```python
from build123d import *

# Parameters (mm, degrees)
BOSS_EXTRUDE1_DEPTH = 50
SKETCH2_W           = 100
SKETCH2_H           = 5
BOSS_EXTRUDE2_DEPTH = 80


with BuildPart() as part:
    # Sketch1 → Boss-Extrude1 (new body)
    with BuildSketch(Plane(origin=(0, 0, 0), x_dir=(1, 0, 0), z_dir=(0, 1, 0))):
        Polygon((0, 0), (490, 0), (490, 20), (420, 20), (420, 170), (400, 170), (400, 20), (310, 20), (310, 170), (290, 170), (290, 20), (200, 20), (200, 170), (180, 170), (180, 20), (90, 20), (90, 170), (70, 170), (70, 20), (0, 20), align=None)
    extrude(amount=BOSS_EXTRUDE1_DEPTH)

    # Sketch2 → Boss-Extrude2 (add)
    with BuildSketch(Plane.XY):
        with Locations((50, 2.5)):
            Rectangle(SKETCH2_W, SKETCH2_H)
    extrude(amount=BOSS_EXTRUDE2_DEPTH)


solid = part.part
```
Read the model definition and answer for the solid it produces. Units are mm, in the model's axes. A direction names the side the tool comes from. Give positions to 0.01 mm unless a question says otherwise; leave off trailing zeros. Write each loop counter-clockwise with the first axis right and the second up, starting at its lowest first coordinate (ties: lowest second). Pieces come first, ordered by that corner, then holes. Notation, with made-up numbers: M -20.5,14.5 L -1.5,14.5 A16 ccw -1.5,39.5 Z; hole C -31,68.25 d9. An arc over 180 degrees is marked long. Put each result on its own line as item: value. Start each with the question number.
1. Consider line 1 along X through (y, z) = (27, -58.5); line 2 along Z through (x, y) = (94, 24.5); line 3 along Z through (x, y) = (24, 4). Determine where each line is inside the solid, lowest interval first.
2. The part is cut by section D-D, the plane z = 56.5. Give the vertices of the cut face in (x, y), and give its area (3 significant figures).
3. For a pull along X with two mould halves and no side action, classify faces 4 (the flat face through (0, 19, -4)), 5 (the flat face through (90, 25, -94)), 6 (the flat face through (187, 0, -47)) as released by +X, released by -X, zero draft, split by the parting line, or undercut.
4. The part is cut by section C-C, the plane x = 186. Give the vertices of the cut face in (y, z).
5. Which of the six approach directions +Z, -Z, +X, -X, +Y, -Y give full straight-line access (tool end or side, diameter ignored) to faces 1 (the flat face through (246, 25, -20)), 2 (the flat face through (70, 25, -96)), 3 (the flat face through (49, 5, 39))?
6. Each of these flat-tipped pins is pushed along its axis until it touches: pin 1 Ø24 at (x, z) = (74, 58) entering from +Y; pin 2 Ø25 at (x, y) = (130.5, 12.5) entering from -Z; pin 3 Ø12 at (y, z) = (25, -29.5) entering from -X. Where does it stop, or does it pass through?
7. The part is cut by section B-B, the plane y = 41.5. Give the vertices of the cut face in (x, z).
8. The part is cut by section A-A, the plane z = -80.5. Give the vertices of the cut face in (x, y).
Final values:
1. line 1: x = 70 to 90, 180 to 200, 290 to 310, 400 to 420
1. line 2: z = -20 to 0
1. line 3: z = -20 to 80
2. outline: M 0,0 L 100,0 L 100,5 L 0,5 Z
2. area: 500 mm²
3. face 4: released by -X
3. face 5: undercut
3. face 6: zero draft
4. outline: M 0,-170 L 50,-170 L 50,0 L 0,0 Z
5. face 1: -Z, +Y, -Y
5. face 2: -Z, -X, +Y, -Y
5. face 3: +Z, +X, -X, +Y
6. pin 1: stops at y = 5
6. pin 2: stops at z = -20
6. pin 3: stops at x = 70
7. outline: M 0,-20 L 70,-20 L 70,-170 L 90,-170 L 90,-20 L 180,-20 L 180,-170 L 200,-170 L 200,-20 L 290,-20 L 290,-170 L 310,-170 L 310,-20 L 400,-20 L 400,-170 L 420,-170 L 420,-20 L 490,-20 L 490,0 L 0,0 Z
8. outline: M 70,0 L 90,0 L 90,50 L 70,50 Z; M 180,0 L 200,0 L 200,50 L 180,50 Z; M 290,0 L 310,0 L 310,50 L 290,50 Z; M 400,0 L 420,0 L 420,50 L 400,50 Z
